Autodesk Inventor part; units mm, degrees
ref_plane "YZ Plane" through (0, 0, 0) normal (1, 0, 0) x (0, 1, 0)
ref_plane "XZ Plane" through (0, 0, 0) normal (0, 1, 0) x (-1, 0, 0)
ref_plane "XY Plane" through (0, 0, 0) normal (0, 0, 1) x (1, 0, 0)
sketch "Sketch1" plane through (0, 0, 0) normal (0, 0, 1) x (1, 0, 0)
  line L0 (-101.6, -22.225) -> (101.6, -22.225)
  line L1 (101.6, -22.225) -> (101.6, 22.225)
  line L2 (101.6, 22.225) -> (-101.6, 22.225)
  line L3 (-101.6, 22.225) -> (-101.6, -22.225)
  line L4 (-19.05, 22.225) -> (-19.05, 3.175)
  arc A0 (-19.05, 3.175) -> (19.05, 3.175) centre (0, 3.175) ccw
  line L5 (19.05, 3.175) -> (19.05, 22.225)
  line L6 (-50.8, 15.875) -> (-44.45, 15.875)
  line L7 (-44.45, 15.875) -> (-44.45, 9.525)
  line L8 (-44.45, 9.525) -> (-50.8, 9.525)
  line L9 (-50.8, 9.525) -> (-50.8, 15.875)
  line L10 (44.45, 15.875) -> (50.8, 15.875)
  line L11 (50.8, 15.875) -> (50.8, 9.525)
  line L12 (50.8, 9.525) -> (44.45, 9.525)
  line L13 (44.45, 9.525) -> (44.45, 15.875)
  line L14 (-50.8, 3.175) -> (-44.45, 3.175)
  line L15 (-44.45, 3.175) -> (-44.45, -3.175)
  line L16 (-44.45, -3.175) -> (-50.8, -3.175)
  line L17 (-50.8, -3.175) -> (-50.8, 3.175)
  line L18 (44.45, 3.175) -> (50.8, 3.175)
  line L19 (50.8, 3.175) -> (50.8, -3.175)
  line L20 (50.8, -3.175) -> (44.45, -3.175)
  line L21 (44.45, -3.175) -> (44.45, 3.175)
  line L22 (-50.8, -9.525) -> (-44.45, -9.525)
  line L23 (-44.45, -9.525) -> (-44.45, -15.875)
  line L24 (-44.45, -15.875) -> (-50.8, -15.875)
  line L25 (-50.8, -15.875) -> (-50.8, -9.525)
  line L26 (44.45, -9.525) -> (50.8, -9.525)
  line L27 (50.8, -9.525) -> (50.8, -15.875)
  line L28 (50.8, -15.875) -> (44.45, -15.875)
  line L29 (44.45, -15.875) -> (44.45, -9.525)
  point P0 (0, 0)
  point P1 (-101.6, 0)
  point P2 (0, 22.225)
  dimension "d0" = 203.2
  dimension "d1" = 44.45
  dimension "d2" = 6.35
  dimension "d3" = 44.45
  dimension "d4" = 6.35
  dimension "d7" = 95.25
  dimension "d10" = 12.7
  dimension "d13" = 19.05
  dimension "d14" = 19.05
extrude "Extrusion1" add sketch "Sketch1" along normal blind 6.35 contours L3 L2 L4 A0 L5 L1 L0
sketch "Sketch2" plane through (0, 0, 6.35) normal (0, 0, 1) x (1, 0, 0)
  line L0 (101.6, -22.225) -> (-101.6, -22.225)
  point P0 (0, 0)
  point P1 (-65.0875, 3.175)
  point P2 (65.0875, 3.175)
  dimension "d18" = 65.0875
  dimension "d26" = 130.175
  dimension "d27" = 25.4
hole "Hole1" at (-65.0875, 3.175, 6.35) at (65.0875, 3.175, 6.35) direction (0, 0, -1) diameter 3.81 end through all
properties part number "acrylic kinect bracket - kinect plate"
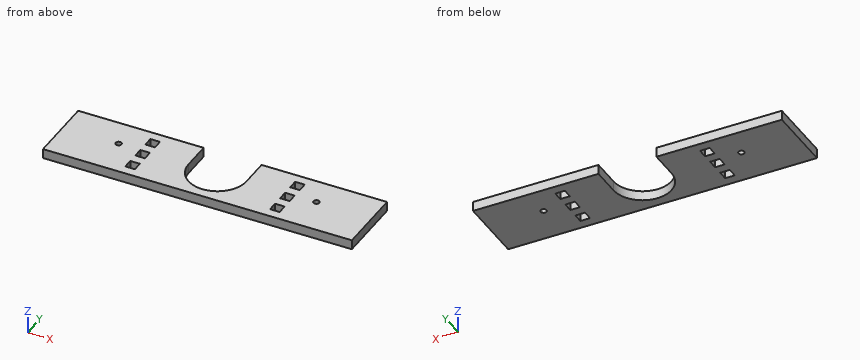
Verification items for the finished model (mm, model axes). Round coordinates to 2 decimals unless told otherwise and drop trailing zeros. Write each loop counter-clockwise with the first axis right and the second up, starting at its lowest first coordinate (ties: lowest second). Pieces come first, ordered by that corner, then holes.
1. Section check B-B on y = -11.5. Enter the section's corners in (x, z).
2. Scan lines: L1, parallel to X at y = 7, z = 0.75; L2, parallel to X at y = -10, z = 3; L3, parallel to X at y = 4.5, z = 0.5. Record each from-to range of solid material in increasing order.
3. Section check A-A on z = 4. State how many separate pieces and enclosed holes the cut face has, plus the area to 3 significant figures.
4. Section check C-C on x = 0. Enter the section's corners in (y, z) (3 decimals), plus the area to 3 significant figures.
5. Gauge pin test, flat end, axial feed: P1, Ø1.5, axis at x = -9, z = 4.5, coming from the +Y side. Record the tip position at first contact, or that the pin passes through.
Answer:
1. outline: (-101.6, 0) - (-50.8, 0) - (-50.8, 6.35) - (-101.6, 6.35) - close; (-44.45, 0) - (-12.15, 0) - (-12.15, 6.35) - (-44.45, 6.35) - close; (12.15, 0) - (44.45, 0) - (44.45, 6.35) - (12.15, 6.35) - close; (50.8, 0) - (101.6, 0) - (101.6, 6.35) - (50.8, 6.35) - close
2. L1: x = -101.6 to -19.05, 19.05 to 101.6
2. L2: x = -101.6 to -50.8, -44.45 to -13.76, 13.76 to 44.45, 50.8 to 101.6
2. L3: x = -101.6 to -66.46, -63.72 to -19.05, 19.05 to 63.72, 66.46 to 101.6
3. separate pieces: 1
3. enclosed holes: 8
3. area: 7,470 mm2
4. outline: (-22.225, 0) - (-15.875, 0) - (-15.875, 6.35) - (-22.225, 6.35) - close
4. area: 40.3 mm2
5. P1: stops at y = -13.19
